Can you work these out from the model? Positions are in its coordinate system, mm. Face numbers are marked on the shaded views. A direction names the side the tool comes from. Give positions to 0.01 mm unless a question says otherwise; leave off trailing zeros. Order: outer loops, then holes, each group sorted by start corner. A loop starts at its lowest first (then second) coordinate and runs counter-clockwise, first axis right, second up. Notation, with made-up numbers: (-29.5, 2) - (23.5, 2) arc R25 ccw to (23.5, 29) - close; hole circle Ø3 at (24.25, 36.25). An arc over 180 degrees is marked (long way). Write each question's results on one line, items separated by ' | '. Start each with the question number.
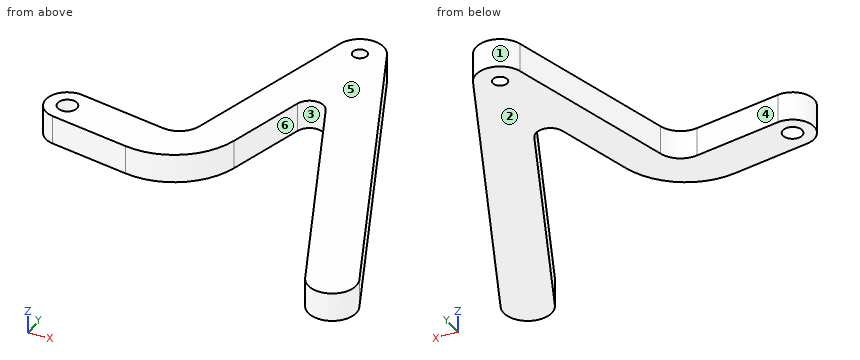
Autodesk Inventor part; units mm, degrees
ref_plane "YZ Plane" through (0, 0, 0) normal (1, 0, 0) x (0, 1, 0)
ref_plane "XZ Plane" through (0, 0, 0) normal (0, 1, 0) x (-1, 0, 0)
ref_plane "XY Plane" through (0, 0, 0) normal (0, 0, 1) x (1, 0, 0)
sketch "Sketch1" plane through (0, 0, 0) normal (0, 0, 1) x (1, 0, 0)
  circle A0 centre (0, 0) radius 2
  arc A1 (0.7814, 4.4316) -> (-0.7814, -4.4316) centre (0, 0) ccw
  arc A2 (44.5957, 41.9696) -> (35.1896, 41.3639) centre (40, 40) ccw
  line L0 (44.5957, 41.9696) -> (74.5957, -28.0304)
  arc A3 (65.4043, -31.9696) -> (74.5957, -28.0304) centre (70, -30) ccw
  circle A4 centre (40, 40) radius 1.5
  line L1 (0, 0) -> (46.8621, 0) construction
  line L2 (65.4043, -31.9696) -> (43.0454, 20.2011)
  line L3 (0.7814, 4.4316) -> (19.1318, 1.196)
  arc A5 (19.1318, 1.196) -> (24.8104, 4.7561) centre (20, 6.12) ccw
  line L4 (24.8104, 4.7561) -> (35.1896, 41.3639)
  line L5 (-0.7814, -4.4316) -> (15.6896, -7.3359)
  arc A6 (15.6896, -7.3359) -> (32.7255, 3.3446) centre (18.2943, 7.4362) ccw
  line L6 (32.7255, 3.3446) -> (37.4017, 19.8377)
  arc A7 (43.0454, 20.2011) -> (37.4017, 19.8377) centre (40.288, 19.0194) ccw
  dimension "d0" = 4
  dimension "d1" = 3
  dimension "d2" = 4.5
  dimension "d5" = 40
  dimension "d6" = 5
  dimension "d8" = 10
  dimension "d9" = 40
  dimension "d10" = 30
  dimension "d11" = 70
  dimension "d12" = 10
  dimension "d13" = 20
  dimension "d14" = 8
  dimension "d15" = 5
  dimension "d16" = 15
  dimension "d17" = 3
extrude "Extrusion1" add sketch "Sketch1" along normal blind 6
properties part number "Leg3"
Q1. Will these pins go through, and if not, where does the flat tip stop? P1, Ø1.5, axis at y = 3, z = 3.5, coming from the +X side; P2, Ø1.5, axis at x = 24.5, z = 1, coming from the -Y side; P3, Ø1, axis at x = 10, z = 4, coming from the -Y side.
Q2. If we section it at C-C (x = 40): Please give me the cut outline in (y, z), plus the area to 3 significant figures.
Q3. If we section it at B-B (y = 40): Please give me the cut outline in (x, z), plus the area to 3 significant figures.
Q4. Which directions (+Z, -Z, +X, -X, +Y, -Y) give clear straight access to the entire face, cutting with the end or side of a thin tool? Please do the marked faces 4, 5 and 6.
Q5. Thinking about a two-plate mould opening in X: for the marked faces 1, 2 and 3, which applies, released by +X, released by -X, zero draft, split by the parting line, or undercut?
Q6. If we section it at D-D (y = 0): Please give me the cut outline in (x, z), plus the area to 3 significant figures.
Q7. If we section it at A-A (z = 1.9): Please give me the cut outline in (x, y), plus the area to 3 significant figures.
Q8. If I drill on probe 1 along Y at (x, z) = (40, 2); probe 2 along X at (y, z) = (-2.5, 3.9); probe 3 along X at (y, z) = (19, 1.1), over which ranges is the centre line in solid material (lowest first)? Write a range as from..to.
Findings below:
1) P1: stops at x = 61.62 | P2: stops at y = -6.54 | P3: stops at y = -6.42
2) outline: (22.01, 0) - (38.5, 0) - (38.5, 6) - (22.01, 6) - close; (41.5, 0) - (45, 0) - (45, 6) - (41.5, 6) - close | area: 120 mm2
3) outline: (34.8, 0) - (38.5, 0) - (38.5, 6) - (34.8, 6) - close; (41.5, 0) - (45.44, 0) - (45.44, 6) - (41.5, 6) - close | area: 45.8 mm2
4) face 4: +Z, -Z, +Y | face 5: +Z, +X, -X, +Y, -Y | face 6: +Z, -Z, -Y
5) face 1: split by the parting line | face 2: zero draft | face 3: undercut
6) outline: (-4.5, 0) - (-2, 0) - (-2, 6) - (-4.5, 6) - close; (2, 0) - (31.32, 0) - (31.32, 6) - (2, 6) - close; (51.7, 0) - (62.58, 0) - (62.58, 6) - (51.7, 6) - close | area: 256 mm2
7) outline: (-0.78, -4.43) - (15.69, -7.34) arc R15 ccw to (32.73, 3.34) - (37.4, 19.84) arc R3 cw to (43.05, 20.2) - (65.4, -31.97) arc R5 ccw to (74.6, -28.03) - (44.6, 41.97) arc R5 ccw to (35.19, 41.36) - (24.81, 4.76) arc R5 cw to (19.13, 1.2) - (0.78, 4.43) arc R4.5 ccw to start; hole circle Ø4 at (0, 0); hole circle Ø3 at (40, 40) | area: 1,390 mm2
8) probe 1: y = 22.01..38.5, 41.5..45 | probe 2: x = -3.74..29.53, 52.77..63.65 | probe 3: x = 28.85..37.16, 43.56..54.44
